```python
from build123d import *

# Parameters (mm, degrees)
SKETCH_1_R      = 2.25
SKETCH_1_R_2    = 1.5
EXTRUDE_1_DEPTH = 5


with BuildPart() as part:
    # 草图1 → 凸台-拉伸1 (new body)
    with BuildSketch(Plane.XY):
        Polygon((0, 0), (150, 0), (150, 367), (122, 367), (122, 400), (112, 400), (112, 367), (75, 367), (38, 367), (38, 400), (28, 400), (28, 367), (0, 367), align=None)
        with Locations((30, 42)):
            Circle(SKETCH_1_R, mode=Mode.SUBTRACT)
        with Locations((120, 42)):
            Circle(SKETCH_1_R, mode=Mode.SUBTRACT)
        with Locations((30, 350)):
            Circle(SKETCH_1_R, mode=Mode.SUBTRACT)
        with Locations((120, 350)):
            Circle(SKETCH_1_R, mode=Mode.SUBTRACT)
        with Locations((25, 50)):
            Circle(SKETCH_1_R_2, mode=Mode.SUBTRACT)
        with Locations((125, 50)):
            Circle(SKETCH_1_R_2, mode=Mode.SUBTRACT)
        with Locations((40, 150)):
            Circle(SKETCH_1_R_2, mode=Mode.SUBTRACT)
        with Locations((125, 150)):
            Circle(SKETCH_1_R_2, mode=Mode.SUBTRACT)
        with Locations((55, 32.5)):
            Circle(SKETCH_1_R, mode=Mode.SUBTRACT)
        with Locations((95, 32.5)):
            Circle(SKETCH_1_R, mode=Mode.SUBTRACT)
    extrude(amount=EXTRUDE_1_DEPTH)


solid = part.part
```
Can you work these out from the model? Positions are in its coordinate system, mm. Coordinates: 2 decimals unless noted, no trailing zeros. Order: outer loops, then holes, each group sorted by start corner. A loop starts at its lowest first (then second) coordinate and runs counter-clockwise, first axis right, second up.
1. I'm going to push flat-ended pins straight in: pin 1 (1 mm diameter, centred on x = 62, z = 1, fed in from +Y); pin 2 (1.5 mm diameter, centred on y = 383.5, z = 2.5, fed in from -X); pin 3 (1.5 mm diameter, centred on y = 383, z = 3, fed in from +X). Where does each tip first touch, or does it pass through?
2. I need wall thicknesses on line 1 (Y direction, x = 125, z = 1.6); line 2 (X direction, y = 150, z = 3.4); line 3 (X direction, y = 377, z = 1.45). Which ranges of each line are inside material? Lowest first, please.
3. If we section it at B-B (x = 65.5): Please give me the cut outline in (y, z).
4. If we section it at A-A (z = 3.2): Give the number of separate pieces and of enclosed holes in the cut face, then the cut area to 3 significant figures.
Entries:
1. pin 1: stops at y = 367
1. pin 2: stops at x = 28
1. pin 3: stops at x = 122
2. line 1: y = 0 to 48.5, 51.5 to 148.5, 151.5 to 367
2. line 2: x = 0 to 38.5, 41.5 to 123.5, 126.5 to 150
2. line 3: x = 28 to 38, 112 to 122
3. outline: (0, 0) - (367, 0) - (367, 5) - (0, 5) - close
4. separate pieces: 1
4. enclosed holes: 10
4. area: 55,600 mm2
